Input: dimensioned drawing with shaded views. Units: mm. Origin: part minimum x, y, z. A direction names the side the tool comes from. Round coordinates to 2 decimals unless told otherwise and drop trailing zeros. Order: outer loops, then holes, each group sorted by start corner. A loop starts at its lowest first (then second) coordinate and runs counter-clockwise, first axis right, second up. Notation, with made-up numbers: M 51.25,21.5 L 63.25,21.5 A14 cw 63.25,48.5 Z; hole C 71.5,49 d5. An arc over 180 degrees is marked long. Use one line per item in the form item = value. Start each with the question number.
Q1. Pull-direction query (Z, two-part tool) for the marked faces 1, 2 and 3; classes: pulls with the +Z half, pulls with the -Z half, needs draft (parallel to the pull), parting line crosses it, or undercut.
Q2. Section A-A (y = 16.5). Return the cut outline in (x, z).
Q3. Section D-D (x = 7.5). Return the cut outline in (y, z).
Q4. Section C-C (z = 10). Return the cut outline in (x, y).
Q5. Contact query for flat-ended pins moving along their axis: pin 1 (11 mm diameter, centred on x = 24.5, y = 8, fed in from -Z); pin 2 (1 mm diameter, centred on x = 46.5, z = 30.5, fed in from +Y). Output: stop coordinate, or through.
Q6. Reachability of the marked faces 4 and 5 from +Z, -Z, +X, -X, +Y, -Y: full face, straight path, thin tool, end or side. Return the list, or none.
Q7. Material intervals for probe 1 along X at (y, z) = (21.5, 46); probe 2 along Z at (x, y) = (51.5, 20); probe 3 along Y at (x, z) = (31, 7.5), sorted ascending.
Q8. Section B-B (x = 15.5). Return the cut outline in (y, z), plus the area to 3 significant figures.
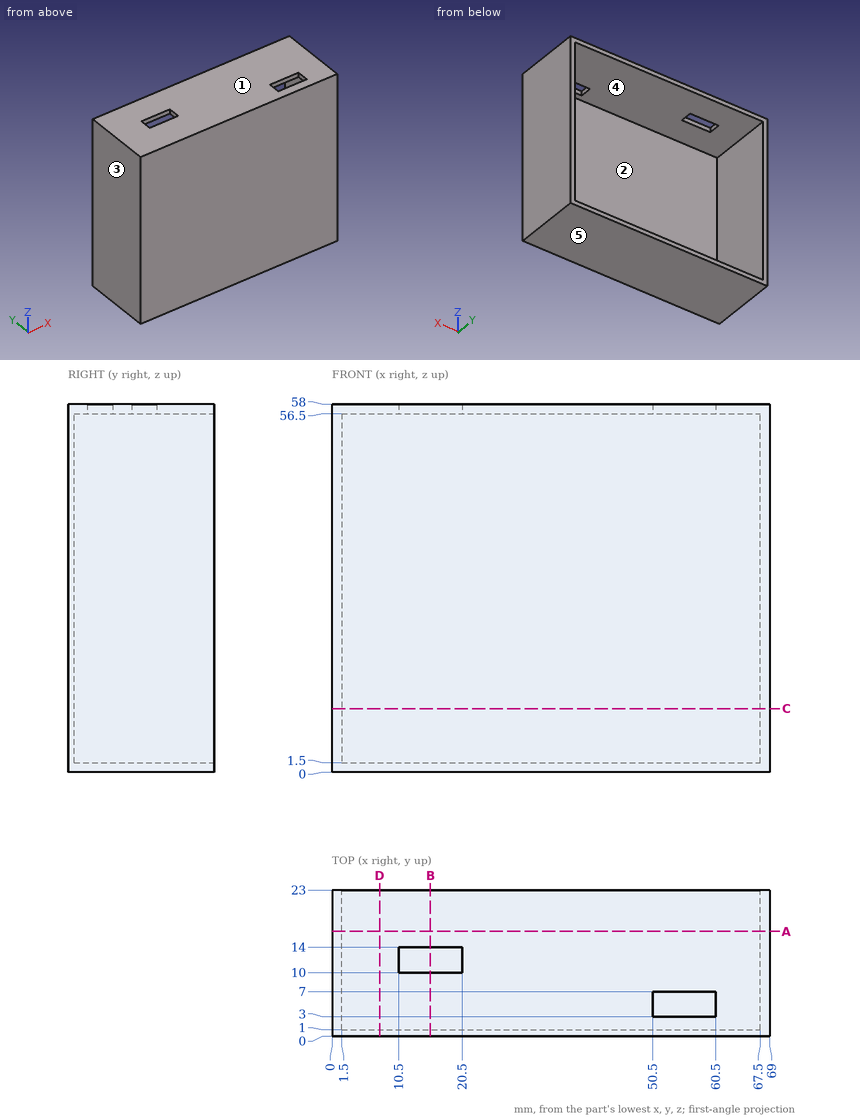
Results list:
q1.face_1 = pulls with the +Z half
q1.face_2 = undercut
q1.face_3 = needs draft
q2.outline = M 0,0 L 69,0 L 69,58 L 0,58 Z; hole M 1.5,1.5 L 67.5,1.5 L 67.5,56.5 L 1.5,56.5 Z
q3.outline = M 0,0 L 23,0 L 23,1.5 L 1,1.5 L 1,56.5 L 23,56.5 L 23,58 L 0,58 Z
q4.outline = M 0,0 L 69,0 L 69,23 L 67.5,23 L 67.5,1 L 1.5,1 L 1.5,23 L 0,23 Z
q5.pin_1 = 0
q5.pin_2 = 1
q6.face_4 = +Y
q6.face_5 = -Z, +X, -X, +Y, -Y
q7.probe_1 = 0 to 1.5, 67.5 to 69
q7.probe_2 = 0 to 1.5, 56.5 to 58
q7.probe_3 = 0 to 1
q8.outline = M 0,0 L 23,0 L 23,1.5 L 1,1.5 L 1,56.5 L 10,56.5 L 10,58 L 0,58 Z; M 14,56.5 L 23,56.5 L 23,58 L 14,58 Z
q8.area = 118 mm2
